The listing builds one solid part. Answer for the finished solid, in the listing's coordinates (mm). Coordinates: 2 decimals unless noted, no trailing zeros. Loops run counter-clockwise (first coordinate to the right, second up) from the corner with the lowest first, then second, coordinate; pieces in that order, holes last. Notation, with made-up numbers: M 19.5,-37.75 L 50.5,-37.75 A20 cw 50.5,-23.75 Z; hole C 14,-37 d8. An arc over 180 degrees is marked long. Return JSON: item names as keys, results as strings. Group by question number.
1. Given P1, Ø3, axis at x = 2, y = 2, coming from the -Z side; P2, Ø1.5, axis at x = 3.5, y = 2.5, coming from the +Z side; P3, Ø3, axis at x = 10.5, y = 3, coming from the +Z side, each flat-ended and moving along its own axis, determine where each tip first touches the part or whether it passes through.
2. Section C-C (x = 11) is taken. Write down the section's boundary in (y, z).
3. Section B-B (x = -10.75) is taken. Write down the section's boundary in (y, z), then the cut area to 3 significant figures.
4. Straight lines are drawn through the part: L1, parallel to Z at x = 0, y = 3.15; L2, parallel to X at y = 2.8, z = 120; L3, parallel to X at y = 1.7, z = 0. For each, find the intervals that lie inside material, in ascending order. Write a range as from..to.
5. Section A-A (y = 2.8) is taken. Write down the section's boundary in (x, z), then the cut area to 3 significant figures.
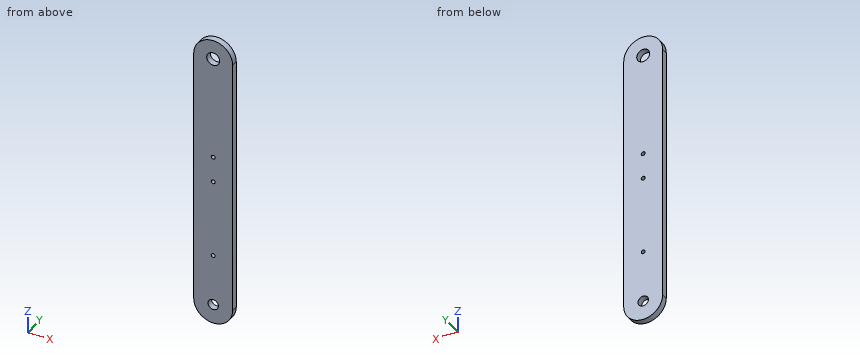
Autodesk Inventor part; units mm, degrees
ref_plane "YZ Plane" through (0, 0, 0) normal (1, 0, 0) x (0, 1, 0)
ref_plane "XZ Plane" through (0, 0, 0) normal (0, 1, 0) x (-1, 0, 0)
ref_plane "XY Plane" through (0, 0, 0) normal (0, 0, 1) x (1, 0, 0)
sketch "Sketch1" plane through (0, 0, 0) normal (0, 1, 0) x (-1, 0, 0)
  circle A0 centre (0, 0) radius 4
  circle A1 centre (0, 200) radius 15
  circle A2 centre (0, 200) radius 5
  circle A3 centre (0, 0) radius 15
  line L0 (15, 200) -> (15, 0)
  line L1 (-15, 200) -> (-15, 0)
  line L2 (0, 160) -> (0, 110) construction
  line L3 (4, 160) -> (4, 110)
  line L4 (-4, 110) -> (-4, 160)
  arc A4 (4, 160) -> (-4, 160) centre (0, 160) ccw
  arc A5 (-4, 110) -> (4, 110) centre (0, 110) ccw
  line L5 (0, -61) -> (0, 261)
  line L6 (4, 90) -> (4, 40)
  arc A6 (4, 90) -> (-4, 90) centre (0, 90) ccw
  line L7 (-4, 40) -> (-4, 90)
  arc A7 (-4, 40) -> (4, 40) centre (0, 40) ccw
  circle A8 centre (0, 175) radius 1.5
  circle A9 centre (0, 100) radius 1.5
  circle A10 centre (0, 120) radius 1.5
  circle A11 centre (0, 40) radius 1.5
  point P0 (0, 135)
  point P1 (-7, 0)
  point P2 (7, 0)
  point P3 (0, 121.5)
  point P4 (0, 118.5)
  dimension "d0" = 8
  dimension "d1" = 30
  dimension "d2" = 200
  dimension "d3" = 10
  dimension "d4" = 30
  dimension "d16" = 8
  dimension "d18" = 50
  dimension "d20" = 14
  dimension "d21" = 7
  dimension "d31" = 65
  dimension "d34" = 70
  dimension "d39" = 40
  dimension "d40" = 40
  dimension "d41" = 75
  dimension "d44" = 3
  dimension "d45" = 3
  dimension "d46" = 3
  dimension "d47" = 25
  dimension "d48" = 3
  dimension "d50" = 40
  dimension "d51" = 100
  dimension "d52" = 120
extrude "Extrusion1" add sketch "Sketch1" along normal blind 5 contours A0 L5 A3 | A0 L5 A3 | L5 A7 L6 A6 A9 A5 L3 A4 A8 A1 L0 A3 | A3 L1 A1 L5 A8 A4 L4 A5 A9 A6 L7 A7 | A7 L7 A6 L5 A11 | L5 A11 A6 L6 A7 | A1 L5 A2 | A1 L5 A2 | A8 L5 | L5 A8 | L5 A10 A5 L4 A4 | A4 L3 A5 L5 A10
properties part number "Canh_Tay_1" material "Nylon 6/6"
Worked out:
{
 "1": {"P1": "z = -14.99", "P2": "z = 214.75", "P3": "z = 212"},
 "2": {"outline": "M 0,-10.2 L 5,-10.2 L 5,210.2 L 0,210.2 Z"},
 "3": {"outline": "M 0,-10.46 L 5,-10.46 L 5,210.46 L 0,210.46 Z", "area": "1,100 mm^2"},
 "4": {"L1": "-15..-4, 4..38.5, 41.5..98.5, 101.5..118.5, 121.5..195, 205..215", "L2": "-15..-1.5, 1.5..15", "L3": "-15..-4, 4..15"},
 "5": {"outline": "M -15,0 A15 ccw 15,0 L 15,200 A15 ccw -15,200 Z; hole C 0,200 d10; hole C 0,0 d8; hole C 0,40 d3; hole C 0,100 d3; hole C 0,120 d3", "area": "6,560 mm^2"}
}
